```python
from build123d import *

# Parameters (mm, degrees)
SKETCH1_R           = 5.8
BOSS_EXTRUDE1_DEPTH = 40
SKETCH3_R           = 4.8
CUT_EXTRUDE1_DEPTH  = 39
SKETCH6_R           = 2
CUT_EXTRUDE3_DEPTH  = 41.832340124
CIRPATTERN1_COUNT   = 4
CUT_EXTRUDE4_REACH  = 42.832
SKETCH7_R           = 1.5


with BuildPart() as part:
    # Sketch1 → Boss-Extrude1 (new body)
    with BuildSketch(Plane(origin=(0, 0, 0), x_dir=(1, 0, 0), z_dir=(0, 1, 0))):
        with Locations(Location((0, 0, 0), (0, 0, 270))):
            Circle(SKETCH1_R)
    extrude(amount=BOSS_EXTRUDE1_DEPTH)

    # Sketch3 → Cut-Extrude1 (cut)
    with BuildSketch(Plane.XZ):
        with Locations(Location((0, 0, 0), (0, 0, 270))):
            Circle(SKETCH3_R)
    extrude(amount=-CUT_EXTRUDE1_DEPTH, mode=Mode.SUBTRACT)

    # Sketch6 → Cut-Extrude3 (cut, through all)
    with BuildSketch(Plane.XY):
        with Locations(Location((0, 30, 0), (0, 0, 90))):
            Circle(SKETCH6_R)
    cut_extrude3 = extrude(amount=-CUT_EXTRUDE3_DEPTH, mode=Mode.SUBTRACT)

    # CirPattern1: Cut-Extrude3 ×4 about axis
    cirpattern1_axis = Axis((0, 40, 0), (0, -1, 0))
    for i in range(1, CIRPATTERN1_COUNT):
        add(cut_extrude3.rotate(cirpattern1_axis, i * 360 / CIRPATTERN1_COUNT), mode=Mode.SUBTRACT)

    # Sketch7 → Cut-Extrude4 (cut, up to next)
    with BuildSketch(Plane(origin=(0, 40, 0), x_dir=(1, 0, 0), z_dir=(0, 1, 0)), mode=Mode.PRIVATE) as cut_extrude4_sk1:
        with Locations(Location((0, 0, 0), (0, 0, 270))):
            Circle(SKETCH7_R)
    cut_extrude4_tool1 = extrude(cut_extrude4_sk1.sketch, amount=-CUT_EXTRUDE4_REACH, mode=Mode.PRIVATE) & part.part
    add(cut_extrude4_tool1.solids().sort_by_distance((0, 40, 0))[0], mode=Mode.SUBTRACT)


solid = part.part
```
For this review, take the finished solid that the model builds, in its own axes (mm). A direction names the side the tool comes from. Give positions to 0.01 mm unless a question says otherwise; leave off trailing zeros. Write each loop counter-clockwise with the first axis right and the second up, starting at its lowest first coordinate (ties: lowest second). Pieces come first, ordered by that corner, then holes.
Item 1: Machinability: for faces 4 (the face through (4.05, 19.23, -2.58)), 5 (the face through (0.45, 39.51, 1.43)), which of the approach directions +Z, -Z, +X, -X, +Y, -Y give a long, thin tool a straight path to every point of the face, cutting with its end or side? Answer none if there is none.
Item 2: Take a section at D-D (z = 3.25). Give the boundary of the cut face in (x, y).
Item 3: Take a section at A-A (x = 0). Give the boundary of the cut face in (y, z).
Item 4: Wall thickness on probe 1 along Z at (x, y) = (0, 27.5); probe 2 along Y at (x, z) = (4.9, 0); probe 3 along Y at (x, z) = (-4, 1.75): over which ranges is each line inside the solid? List them lowest first.
Item 5: Insertion check: P1, Ø3, axis at x = -2.5, z = 1, coming from the -Y side; P2, Ø1.5, axis at x = -2.5, y = 29.5, coming from the -Z side. Each pin has a flat end and moves straight along its axis. Give the tip position at first contact, or say it passes through.
Item 6: Take a section at C-C (y = 28.5). Give the boundary of the cut face in (x, z).
Item 7: Take a section at B-B (z = 0). Give the boundary of the cut face in (x, y).
Item 8: The part is to be moulded in two halves that separate along X. For faces 1 (the face through (1.742, 19.72, 5.532)), 2 (the face through (5, 0, 1)), 3 (the face through (-0.766, 31.847, 5.072)), say which applies: +X half, -X half, draft (parallel to the pull), parting line (faces both ways), or undercut.
Established:
1. face 4: -Y
1. face 5: +Y, -Y
2. outline: (-4.8, 0) - (-3.53, 0) - (-3.53, 39) - (3.53, 39) - (3.53, 0) - (4.8, 0) - (4.8, 40) - (-4.8, 40) - close
3. outline: (0, -5.8) - (28, -5.8) - (28, -4.8) - (0, -4.8) - close; (0, 4.8) - (28, 4.8) - (28, 5.8) - (0, 5.8) - close; (32, -5.8) - (40, -5.8) - (40, -1.5) - (39, -1.5) - (39, -4.8) - (32, -4.8) - close; (32, 4.8) - (39, 4.8) - (39, 1.5) - (40, 1.5) - (40, 5.8) - (32, 5.8) - close
4. probe 1: z = -5.8 to -4.8, 4.8 to 5.8
4. probe 2: y = 0 to 28, 32 to 40
4. probe 3: y = 39 to 40
5. P1: stops at y = 39
5. P2: stops at z = -5.51
6. outline: (-5.65, -1.32) arc R5.8 ccw to (-1.32, -5.65) - (-1.32, -4.61) arc R4.8 cw to (-4.61, -1.32) - close; (-5.65, 1.32) - (-4.61, 1.32) arc R4.8 cw to (-1.32, 4.61) - (-1.32, 5.65) arc R5.8 ccw to start; (1.32, -5.65) arc R5.8 ccw to (5.65, -1.32) - (4.61, -1.32) arc R4.8 cw to (1.32, -4.61) - close; (1.32, 4.61) arc R4.8 cw to (4.61, 1.32) - (5.65, 1.32) arc R5.8 ccw to (1.32, 5.65) - close
7. outline: (-5.8, 0) - (-4.8, 0) - (-4.8, 28) - (-5.8, 28) - close; (-5.8, 32) - (-4.8, 32) - (-4.8, 39) - (-1.5, 39) - (-1.5, 40) - (-5.8, 40) - close; (1.5, 39) - (4.8, 39) - (4.8, 32) - (5.8, 32) - (5.8, 40) - (1.5, 40) - close; (4.8, 0) - (5.8, 0) - (5.8, 28) - (4.8, 28) - close
8. face 1: parting line
8. face 2: draft
8. face 3: undercut
